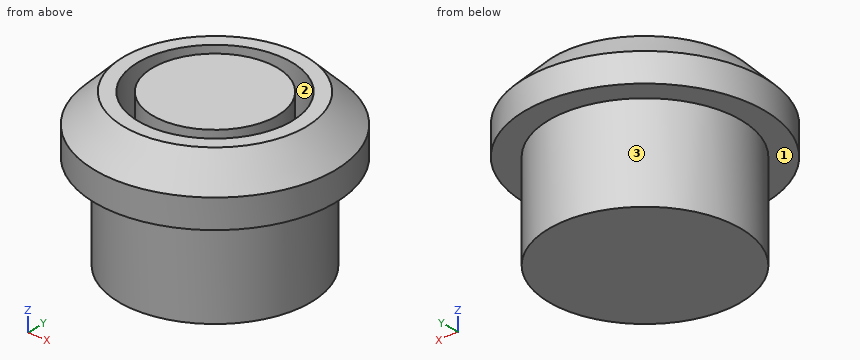
```python
from build123d import *

# Parameters (mm, degrees)
ESQUISSE1_R             = 12.5
BASE_EXTRUSION_DEPTH    = 6
CHANFREIN1_SIZE         = 3
ESQUISSE2_R             = 10
BOSS_EXTRU_1_DEPTH      = 10
ESQUISSE3_R             = 8
ENL_V_MAT_EXTRU_1_DEPTH = 10
ESQUISSE4_R             = 6.5
BOSS_EXTRU_2_DEPTH      = 10


with BuildPart() as part:
    # Esquisse1 → Base-Extrusion (new body)
    with BuildSketch(Plane.XY):
        Circle(ESQUISSE1_R)
    extrude(amount=BASE_EXTRUSION_DEPTH)

    # Chanfrein1
    chanfrein1_edges = [part.edges().sort_by_distance(p)[0] for p in [
        (-12.5, 0, 6),
    ]]
    chamfer(chanfrein1_edges, length=CHANFREIN1_SIZE)

    # Esquisse2 → Boss.-Extru.1 (add)
    with BuildSketch(Plane(origin=(0, 0, 0), x_dir=(-1, 0, 0), z_dir=(0, 0, -1))):
        with Locations(Location((0, 0, 0), (0, 0, 180))):
            Circle(ESQUISSE2_R)
    extrude(amount=BOSS_EXTRU_1_DEPTH)

    # Esquisse3 → Enlèv. mat.-Extru.1 (cut)
    with BuildSketch(Plane.XY.offset(6)):
        Circle(ESQUISSE3_R)
    extrude(amount=-ENL_V_MAT_EXTRU_1_DEPTH, mode=Mode.SUBTRACT)

    # Esquisse4 → Boss.-Extru.2 (add)
    with BuildSketch(Plane.XY.offset(-4)):
        Circle(ESQUISSE4_R)
    extrude(amount=BOSS_EXTRU_2_DEPTH)


solid = part.part
```
CAD build for the part. Positions are in the model's coordinates, mm. Face numbers are marked on the shaded views. Coordinates: 2 decimals unless noted, no trailing zeros. Loops run counter-clockwise (first coordinate to the right, second up) from the corner with the lowest first, then second, coordinate; pieces in that order, holes last. Notation, with made-up numbers: (83, 54) - (114, 54) arc R14 ccw to (114, 66) - close; hole circle Ø9 at (79.5, 31). An arc over 180 degrees is marked (long way). Use CSV: the item, a comma, the result in double quotes. Start each with the question number.
Q1. Cut at D-D, the plane z = 0.75. List the corners of the cut face in (x, y).
Q2. Two-plate mould, pull along X, no slides. Class the marked faces 1, 2 and 3: +X half, -X half, draft (parallel to the pull), parting line (faces both ways), or undercut.
Q3. Drop flat-ended pins along their axis: P1, Ø6, axis at x = 8, z = 3.5, coming from the -Y side; P2, Ø5, axis at y = -3.5, z = -6.5, coming from the +X side; P3, Ø2, axis at x = -4, z = -7.5, coming from the +Y side. Give the stop position or say it passes through.
Q4. Cut at B-B, the plane y = 0. List the corners of the cut face in (x, z), then the cut area to 3 significant figures.
Q5. Cut at A-A, the plane z = -3.25. List the corners of the cut face in (x, y).
Q6. Probe probe 1 along Y at (x, z) = (0, -1.5); probe 2 along Y at (x, z) = (0, 2.75); probe 3 along X at (y, z) = (-0.75, 1). List the from-to ranges inside material, lowest first. Write a range as from..to.
Here are the results:
1,outline,"circle Ø25 at (0, 0); circle Ø13 at (0, 0); hole circle Ø16 at (0, 0)"
2,face 1,"draft"
2,face 2,"undercut"
2,face 3,"parting line"
3,P1,"y = -11.44"
3,P2,"x = 9.95"
3,P3,"y = 9.54"
4,outline,"(-12.5, 0) - (-10, 0) - (-10, -10) - (10, -10) - (10, 0) - (12.5, 0) - (12.5, 3) - (9.5, 6) - (8, 6) - (8, -4) - (6.5, -4) - (6.5, 6) - (-6.5, 6) - (-6.5, -4) - (-8, -4) - (-8, 6) - (-9.5, 6) - (-12.5, 3) - close"
4,area,"311 mm2"
5,outline,"circle Ø20 at (0, 0); circle Ø13 at (0, 0); hole circle Ø16 at (0, 0)"
6,probe 1,"-10..-8, -6.5..6.5, 8..10"
6,probe 2,"-12.5..-8, -6.5..6.5, 8..12.5"
6,probe 3,"-12.48..-7.96, -6.46..6.46, 7.96..12.48"
